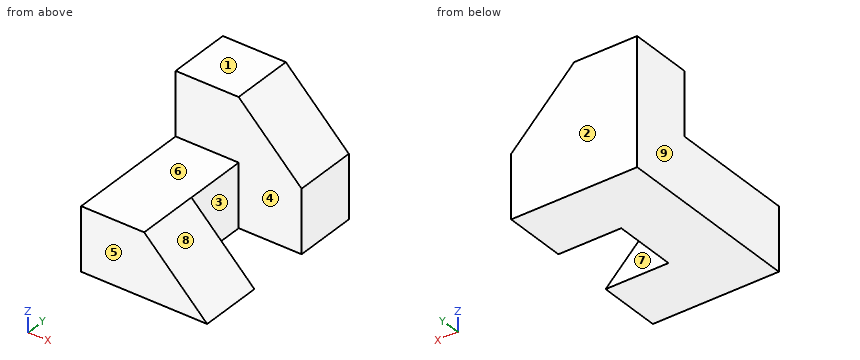
```python
from build123d import *

# Parameters (mm, degrees)
F2_DEPTH = 76.2
F3_DEPTH = 50.8
F4_W     = 25.355122
F4_H     = 25.4
F5_DEPTH = 25.4
F7_DEPTH = 25.4


with BuildPart() as f2:
    # F0 (on Front) → F2 (new body)
    with BuildSketch(Plane.XZ):
        Polygon((0, 25.4), (0, 0), (50.8, 0), (50.8, 25.4), (25.4, 50.8), (0, 50.8), align=None)
    extrude(amount=-F2_DEPTH)

    # F1 (on Right) → F3 (cut)
    with BuildSketch(Plane.YZ):
        Polygon((50.8, 25.4), (50.8, 50.8), (0, 50.8), (0, 25.4), (25.4, 25.4), align=None)
    extrude(amount=F3_DEPTH, mode=Mode.SUBTRACT)

    # F4 (on Top) → F5 (cut)
    with BuildSketch(Plane.XY):
        with Locations((38.122439, 38.1)):
            Rectangle(F4_W, F4_H)
    extrude(amount=F5_DEPTH, mode=Mode.SUBTRACT)

    # F6 (on face) → F7 (cut)
    with BuildSketch(Plane.XZ):
        Polygon((25.4, 25.4), (50.8, 0), (50.8, 25.4), align=None)
    extrude(amount=-F7_DEPTH, mode=Mode.SUBTRACT)


solid = f2.part
```
Build history of the part. All positions in model axes, mm. Face numbers are marked on the shaded views. A direction names the side the tool comes from. Round coordinates to 2 decimals unless told otherwise and drop trailing zeros. Write each loop counter-clockwise with the first axis right and the second up, starting at its lowest first coordinate (ties: lowest second). Pieces come first, ordered by that corner, then holes.
1) Pin check, flat tips, straight feed: pin 1 (10 mm diameter, centred on y = 52.5, z = 30, fed in from -X); pin 2 (1 mm diameter, centred on y = 61, z = 37.5, fed in from +X); pin 3 (3 mm diameter, centred on x = 35, z = 31, fed in from -Y); pin 4 (8 mm diameter, centred on y = 20.5, z = 18, fed in from +X). Stop position of each tip, or through.
2) 3-axis set-ups, long thin cutter, end or side, ignore diameter. For the marked faces 5, 6, 7, 8 and 9: which of +Z, -Z, +X, -X, +Y, -Y reach the whole face in a straight line?
3) Band-saw the part on B-B, the plane z = 20. List the corners of the cut face in (x, y), and give its area (3 significant figures).
4) Band-saw the part on D-D, the plane x = 14.5. List the corners of the cut face in (y, z), and give its area (3 significant figures).
5) Drill centre lines: probe 1 along Y at (x, z) = (39.5, 10); probe 2 along X at (y, z) = (32.5, 17.5); probe 3 along Y at (x, z) = (25.5, 48). Where is each one in solid material? Low to high.
6) Band-saw the part on A-A, the plane x = 33. List the corners of the cut face in (y, z).
7) Mould opens along Y. For the marked faces 1, 2, 3 and 4 say: +Y half, -Y half, draft (parallel to the pull), parting line (faces both ways), or undercut.
8) Band-saw the part on C-C, the plane y = 64. List the corners of the cut face in (x, z), and give its area (3 significant figures).
Ans:
1. pin 1: stops at x = 0
1. pin 2: stops at x = 39.2
1. pin 3: stops at y = 50.8
1. pin 4: stops at x = 36.8
2. face 5: +Z, -Z, +X, -X, -Y
2. face 6: +Z, +X, -X, -Y
2. face 7: +Z, -Z, +X
2. face 8: +Z, +X, -Y
2. face 9: +Z, -Z, -X, +Y, -Y
3. outline: (0, 0) - (30.8, 0) - (30.8, 25.4) - (25.44, 25.4) - (25.44, 50.8) - (50.8, 50.8) - (50.8, 76.2) - (0, 76.2) - close
3. area: 2,720 mm2
4. outline: (0, 0) - (76.2, 0) - (76.2, 50.8) - (50.8, 50.8) - (50.8, 25.4) - (0, 25.4) - close
4. area: 2,580 mm2
5. probe 1: y = 0 to 25.4, 50.8 to 76.2
5. probe 2: x = 0 to 25.44
5. probe 3: y = 50.8 to 76.2
6. outline: (0, 0) - (25.4, 0) - (25.4, 17.8) - (0, 17.8) - close; (50.8, 0) - (76.2, 0) - (76.2, 43.2) - (50.8, 43.2) - close
7. face 1: draft
7. face 2: +Y half
7. face 3: undercut
7. face 4: undercut
8. outline: (0, 0) - (50.8, 0) - (50.8, 25.4) - (25.4, 50.8) - (0, 50.8) - close
8. area: 2,260 mm2
